Print and shaded views of the part. All mm, measured from the part's lowest x, y and z. A direction names the side the tool comes from. Round coordinates to 2 decimals unless told otherwise and drop trailing zeros. Write each loop counter-clockwise with the first axis right and the second up, starting at its lowest first coordinate (ties: lowest second). Pieces come first, ordered by that corner, then holes. Notation, with made-up numbers: (81, -12.75) -> (106, -12.75) arc R34 cw to (106, 20.25) -> close; hole circle Ø1 at (5.25, 64.25). An arc over 180 degrees is marked (long way). Use CSV: the item, a comma, the result in double quotes. Start each with the question number.
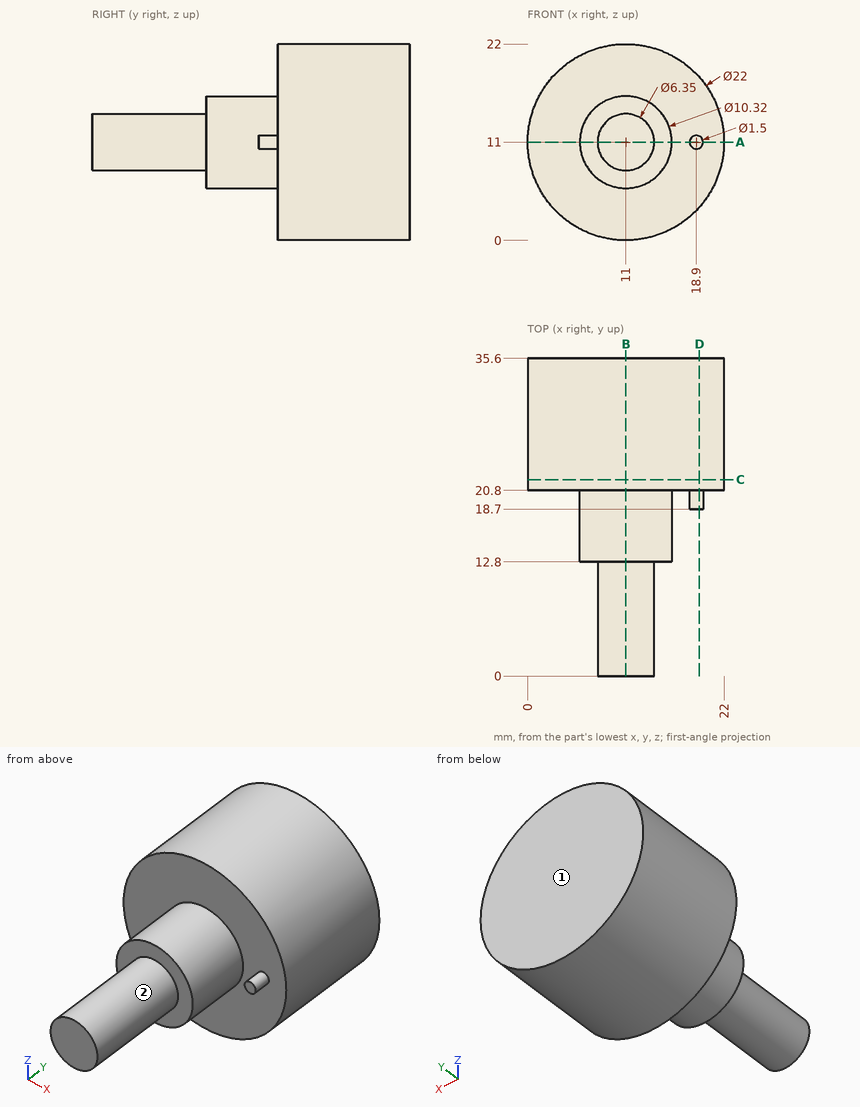
1. Band-saw the part on B-B (x = 11). List the corners of the cut face in (y, z) (3 decimals), then the cut area to 3 significant figures.
2. Band-saw the part on A-A (z = 11). List the corners of the cut face in (x, y) (3 decimals).
3. Band-saw the part on C-C (y = 22). List the corners of the cut face in (x, z), then the cut area to 3 significant figures.
4. Drill centre lines: line 1 along Y through (x, z) = (19.25, 14.75); line 2 along Y through (x, z) = (15.75, 12.5); line 3 along Z through (x, y) = (11.5, 14). Where is each one in solid material? Low to high. Write a range as [from, to].
5. Flat gauge pins, fed straight in: pin 1 (2 mm diameter, centred on y = 29.5, z = 8.5, fed in from +X); pin 2 (1.6 mm diameter, centred on x = 18.5, z = 11, fed in from -Y); pin 3 (3 mm diameter, centred on x = 10.5, z = 4, fed in from -Y). Where does each tip first touch, or does it go through?
6. Band-saw the part on D-D (x = 19.25). List the corners of the cut face in (y, z).
7. Which spindle directions (+Z, -Z, +X, -X, +Y, -Y) get a long thin tool onto all of the face, cutting with end or side? Do the marked faces 1 and 2. Say none if no direction does.
Answers below:
1,outline,"(0, 7.825) -> (12.8, 7.825) -> (12.8, 5.84) -> (20.8, 5.84) -> (20.8, 0) -> (35.6, 0) -> (35.6, 22) -> (20.8, 22) -> (20.8, 16.16) -> (12.8, 16.16) -> (12.8, 14.175) -> (0, 14.175) -> close"
1,area,"489 mm^2"
2,outline,"(0, 20.8) -> (5.84, 20.8) -> (5.84, 12.8) -> (7.825, 12.8) -> (7.825, 0) -> (14.175, 0) -> (14.175, 12.8) -> (16.16, 12.8) -> (16.16, 20.8) -> (18.15, 20.8) -> (18.15, 18.7) -> (19.65, 18.7) -> (19.65, 20.8) -> (22, 20.8) -> (22, 35.6) -> (0, 35.6) -> close"
3,outline,"circle Ø22 at (11, 11)"
3,area,"380 mm^2"
4,line 1,"y = [20.8, 35.6]"
4,line 2,"y = [12.8, 35.6]"
4,line 3,"z = [5.86, 16.14]"
5,pin 1,"stops at x = 21.9"
5,pin 2,"stops at y = 18.7"
5,pin 3,"stops at y = 20.8"
6,outline,"(18.7, 10.34) -> (20.8, 10.34) -> (20.8, 3.72) -> (35.6, 3.72) -> (35.6, 18.28) -> (20.8, 18.28) -> (20.8, 11.66) -> (18.7, 11.66) -> close"
7,face 1,"+Z, -Z, +X, -X, +Y"
7,face 2,"-Y"
